For this review, take the finished solid that the model builds, in its own axes (mm). A direction names the side the tool comes from. Coordinates: 2 decimals unless noted, no trailing zeros. Loops run counter-clockwise (first coordinate to the right, second up) from the corner with the lowest first, then second, coordinate; pieces in that order, holes last. Notation, with made-up numbers: (-23.75, 87) - (9.25, 87) arc R30 cw to (9.25, 115) - close; hole circle Ø2 at (70, -30). An arc over 180 degrees is marked (long way). Use one line per item in the form item = value. Start each with the question number.
1. Add section C-C on x = -7. Give the boundary of the cut face in (y, z).
2. For pin 1 Ø24 at (y, z) = (7, 3) entering from -X, flat-tipped, find the tip position at first contact; note if it passes through.
3. Draft analysis for pull direction Y (two halves, no side actions). For faces 1 (the face through (-28.602, 48.797, -23.859)), 2 (the face through (-73.797, -0.644, -23.859)), 3 (the face through (-15, 0, 0)), state which applies: +Y half, -Y half, draft (parallel to the pull), parting line (faces both ways), or undercut.
4. Add section B-B on x = -63. Give the boundary of the cut face in (y, z).
5. Add section D-D on z = 17.5. Give the boundary of the cut face in (x, y).
6. Add section A-A on z = 0. Give the boundary of the cut face in (x, y).
7. Machinability: for faces 4 (the face through (-45.42, 0.66, -14.985)), 5 (the face through (-17, 1, -25)), which of the approach directions +Z, -Z, +X, -X, +Y, -Y give a long, thin tool a straight path to every point of the face, cutting with its end or side? Answer none if there is none.
8. To check wall thickness, follow probe 1 along Y at (x, z) = (-37, 0); probe 2 along Y at (x, z) = (0, 14.5); probe 3 along X at (y, z) = (7, 3). State the ranges of each line that lie inside material, in increasing order.
```python
from build123d import *

# Parameters (mm, degrees)
SKETCH1_R           = 12.5
BOSS_EXTRUDE1_DEPTH = 25
SKETCH2_R           = 15
CUT_EXTRUDE1_DEPTH  = 60
FILLET1_R           = 4


with BuildPart() as part:
    # Sketch1 → Boss-Extrude1 (new, symmetric)
    with BuildSketch(Plane.XY):
        with BuildLine():
            Line((-75, -50), (75, -50))
            Line((75, -50), (75, -10))
            ThreePointArc((75, -10), (57.426406871, 32.426406871), (15, 50))
            Line((15, 50), (-75, 50))
            Line((-75, 50), (-75, -50))
        make_face()
        Circle(SKETCH1_R, mode=Mode.SUBTRACT)
    extrude(amount=BOSS_EXTRUDE1_DEPTH, both=True)

    # Sketch2 → Cut-Extrude1 (cut)
    with BuildSketch(Plane.ZY.offset(75)):
        Circle(SKETCH2_R)
    extrude(amount=-CUT_EXTRUDE1_DEPTH, mode=Mode.SUBTRACT)

    # Fillet1
    fillet1_edges = [part.edges().sort_by_distance(p)[0] for p in [
        (0, -50, -25),
        (75, -30, -25),
        (57.426406871, 32.426406871, -25),
        (-30, 50, -25),
        (57.426406871, 32.426406871, 25),
        (75, -30, 25),
        (0, -50, 25),
        (-75, 0, 25),
        (-30, 50, 25),
        (-75, 0, -25),
        (75, -50, 0),
        (-75, -50, 0),
        (-75, 50, 0),
    ]]
    fillet(fillet1_edges, radius=FILLET1_R)


solid = part.part
```
Conclusion:
q1.outline = (-50, -21) arc R4 ccw to (-46, -25) - (-10.36, -25) - (-10.36, 25) - (-46, 25) arc R4 ccw to (-50, 21) - close; (10.36, -25) - (46, -25) arc R4 ccw to (50, -21) - (50, 21) arc R4 ccw to (46, 25) - (10.36, 25) - close
q2.pin_1 = -75
q3.face_1 = +Y half
q3.face_2 = draft
q3.face_3 = undercut
q4.outline = (-50, -21) arc R4 ccw to (-46, -25) - (46, -25) arc R4 ccw to (50, -21) - (50, 21) arc R4 ccw to (46, 25) - (-46, 25) arc R4 ccw to (-50, 21) - close; hole circle Ø30 at (0, 0)
q5.outline = (-75, -46) arc R4 ccw to (-71, -50) - (71, -50) arc R4 ccw to (75, -46) - (75, -10) arc R60 ccw to (15, 50) - (-71, 50) arc R4 ccw to (-75, 46) - close; hole circle Ø25 at (0, 0)
q6.outline = (-75, -46) arc R4 ccw to (-71, -50) - (71, -50) arc R4 ccw to (75, -46) - (75, -10) arc R60 ccw to (15, 50) - (-71, 50) arc R4 ccw to (-75, 46) - (-75, 15) - (-15, 15) - (-15, -15) - (-75, -15) - close; hole circle Ø25 at (0, 0)
q7.face_4 = -X
q7.face_5 = -Z, +X, -X, +Y, -Y
q8.probe_1 = -50 to -15, 15 to 50
q8.probe_2 = -50 to -12.5, 12.5 to 50
q8.probe_3 = -15 to -10.36, 10.36 to 72.54
